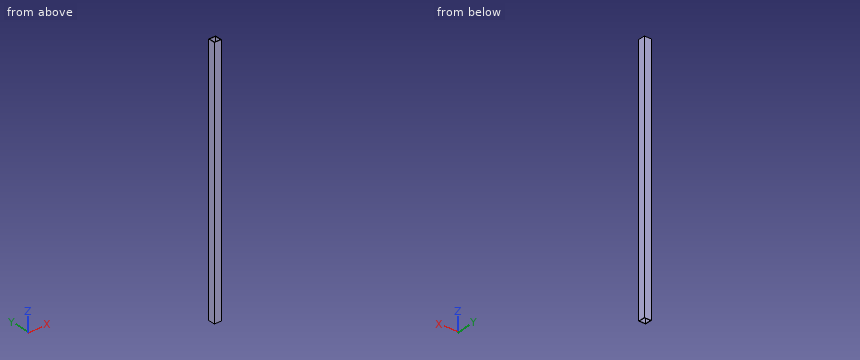
Autodesk Inventor part; units mm, degrees
ref_plane "YZ Plane" through (0, 0, 0) normal (1, 0, 0) x (0, 1, 0)
ref_plane "XZ Plane" through (0, 0, 0) normal (0, 1, 0) x (-1, 0, 0)
ref_plane "XY Plane" through (0, 0, 0) normal (0, 0, 1) x (1, 0, 0)
sketch "Sketch1" plane through (0, 0, 0) normal (0, 0, 1) x (1, 0, 0)
  line L0 (0, 0) -> (25.4, 0)
  line L1 (25.4, 0) -> (25.4, 25.4)
  line L2 (25.4, 25.4) -> (0, 25.4)
  line L3 (0, 25.4) -> (0, 0)
  dimension "d0" = 25.4
  dimension "d1" = 25.4
extrude "Extrusion1" add sketch "Sketch1" along normal blind 939.8
shell "Shell1" thickness 1.5875 removed faces 2 at (8.4667, 16.9333, 0) at (8.4667, 16.9333, 939.8)
properties part number "RearFrameRail" material "Aluminum-6061"
Input: part model. Units: mm. Frame: model coordinates. Round coordinates to 2 decimals unless told otherwise and drop trailing zeros. Write each loop counter-clockwise with the first axis right and the second up, starting at its lowest first coordinate (ties: lowest second). Pieces come first, ordered by that corner, then holes. Notation, with made-up numbers: (-10.75, -0.75) -> (32.25, -0.75) arc R4 cw to (32.25, 3.25) -> close; hole circle Ø11 at (-40, -35). An arc over 180 degrees is marked (long way). Answer as CSV lines item,"result".
1. Section A-A (y = 17.75). Return the cut outline in (x, z), plus the area to 3 significant figures.
Geometry says:
outline,"(0, 0) -> (1.59, 0) -> (1.59, 939.8) -> (0, 939.8) -> close; (23.81, 0) -> (25.4, 0) -> (25.4, 939.8) -> (23.81, 939.8) -> close"
area,"2,980 mm^2"
2. Ray query, L1, parallel to Y at x = 15, z = 879. Return the intervals inside material, ascending. Write a range as [from, to].
Geometry says:
L1,"y = [0, 1.59], [23.81, 25.4]"
3. Section C-C (z = 555.5). Return the cut outline in (x, y), plus the area to 3 significant figures.
Geometry says:
outline,"(0, 0) -> (25.4, 0) -> (25.4, 25.4) -> (0, 25.4) -> close; hole (1.59, 1.59) -> (23.81, 1.59) -> (23.81, 23.81) -> (1.59, 23.81) -> close"
area,"151 mm^2"
4. Contact query for a flat-ended pin moving along its axis: P1, Ø1.5, axis at x = 13, y = 22.5, coming from the -Z side. Output: stop coordinate, or through.
Geometry says:
P1,"passes through"
